```python
from build123d import *

# Parameters (mm, degrees)
SZKIC1_R                        = 5
DODANIE_WYCI_GNI_CIE1_DEPTH     = 18
WYTNIJ_WYCI_GNI_CIE1_DEPTH      = 5
WYTNIJ_WYCI_GNI_CIE1_DEPTH_BACK = 5
WYTNIJ_WYCI_GNI_CIE2_DEPTH      = 5
WYTNIJ_WYCI_GNI_CIE2_DEPTH_BACK = 3
SZKIC3_W                        = 2.5
SZKIC3_H                        = 5.64
WYTNIJ_WYCI_GNI_CIE3_REACH      = 21.339
SZKIC4_R                        = 1.6
WYTNIJ_WYCI_GNI_CIE4_DEPTH      = 2.5


with BuildPart() as part:
    # Szkic1 → Dodanie-wyciągnięcie1 (new body)
    with BuildSketch(Plane.XY):
        Circle(SZKIC1_R)
    extrude(amount=DODANIE_WYCI_GNI_CIE1_DEPTH)

    # Szkic2 → Wytnij-wyciągnięcie1 (cut, two sides: drawn at the far end of the back side and taken through both)
    with BuildSketch(Plane(origin=(0, 0, 0), x_dir=(1, 0, 0), z_dir=(0, 1, 0)).offset(-WYTNIJ_WYCI_GNI_CIE1_DEPTH_BACK)):
        Polygon((-5, -18), (5, -18), (-5, -8), align=None)
    extrude(amount=WYTNIJ_WYCI_GNI_CIE1_DEPTH + WYTNIJ_WYCI_GNI_CIE1_DEPTH_BACK, mode=Mode.SUBTRACT)

    # Szkic3 → Wytnij-wyciągnięcie2 (cut, two sides: drawn at the far end of the back side and taken through both)
    with BuildSketch(Plane(origin=(0, 0, 0), x_dir=(0, 0, -1), z_dir=(1, 0, 0)).offset(-WYTNIJ_WYCI_GNI_CIE2_DEPTH_BACK)):
        with Locations((-3.25, 0)):
            Rectangle(SZKIC3_W, SZKIC3_H)
    extrude(amount=WYTNIJ_WYCI_GNI_CIE2_DEPTH + WYTNIJ_WYCI_GNI_CIE2_DEPTH_BACK, mode=Mode.SUBTRACT)

    # Szkic4 → Wytnij-wyciągnięcie3 (cut, up to next)
    with BuildSketch(Plane(origin=(0, 0, 0), x_dir=(-1, 0, 0), z_dir=(0, 0, -1)), mode=Mode.PRIVATE) as wytnij_wyci_gni_cie3_sk1:
        Circle(SZKIC4_R)
    wytnij_wyci_gni_cie3_tool1 = extrude(wytnij_wyci_gni_cie3_sk1.sketch, amount=-WYTNIJ_WYCI_GNI_CIE3_REACH, mode=Mode.PRIVATE) & part.part
    add(wytnij_wyci_gni_cie3_tool1.solids().sort_by_distance((0, 0, 0))[0], mode=Mode.SUBTRACT)

    # Szkic5 → Wytnij-wyciągnięcie4 (cut)
    with BuildSketch(Plane.XY.offset(2)):
        Polygon((-3, -2.82), (-3, 2.82), (-4.333128401, 0), align=None)
    extrude(amount=WYTNIJ_WYCI_GNI_CIE4_DEPTH, mode=Mode.SUBTRACT)


solid = part.part
```
Design review of the part built by this model. Coordinates are the model's own, in mm. A direction names the side the tool comes from. Give positions to 0.01 mm unless a question says otherwise; leave off trailing zeros. Order: outer loops, then holes, each group sorted by start corner. A loop starts at its lowest first (then second) coordinate and runs counter-clockwise, first axis right, second up. Notation, with made-up numbers: (86.25, -11.75) -> (137.25, -11.75) arc R23 cw to (137.25, 20.25) -> close; hole circle Ø4 at (12, -2). An arc over 180 degrees is marked (long way). Write item = value, one per line. Start each with the question number.
(1) For pin 1 (4 mm diameter, centred on x = -2.5, z = 10, fed in from +Y); pin 2 (3 mm diameter, centred on x = 2, y = 0, fed in from +Z); pin 3 (3.5 mm diameter, centred on x = 0, y = 0, fed in from +Z), all flat-tipped, find the tip position at first contact; note any pin that passes through.
(2) We need section C-C on x = 0. Write out the cut boundary in (y, z).
(3) We need section D-D on z = 4. Write out the cut boundary in (x, y).
(4) For faces 1 (the face through (1, 2.82, 3)), 2 (the face through (1.27, -0.97, 0.99)), 3 (the face through (4.77, 1.5, 6.87)), list the 3-axis set-ups (+Z, -Z, +X, -X, +Y, -Y) from which the entire face can be reached by the end or side of a thin tool; tool diameter is ignored.
(5) We need section A-A on x = 3. Write out the cut boundary in (y, z).
(6) We need section B-B on y = 1. Write out the cut boundary in (x, z).
(7) Mouldability with a two-part tool opening along Z and no side actions: class faces 4 (the face through (2, 0, 0)), 5 (the face through (1, -2.82, 3)), 6 (the face through (0, 0, 4.5)), 7 (the face through (0, 0, 13)) as +Z half, -Z half, draft (parallel to the pull), parting line (faces both ways), or undercut.
(8) To check wall thickness, follow line 1 along Y through (x, z) = (0, 0.95); line 2 along Y through (x, z) = (-2, 3); line 3 along Z through (x, y) = (2, -2.75). State the ranges of each line that lie inside material, in increasing order.
Numbers:
q1.pin_1 = 4.97
q1.pin_2 = 16.5
q1.pin_3 = 14.75
q2.outline = (-5, 0) -> (-1.6, 0) -> (-1.6, 2) -> (-2.82, 2) -> (-2.82, 4.5) -> (2.82, 4.5) -> (2.82, 2) -> (1.6, 2) -> (1.6, 0) -> (5, 0) -> (5, 13) -> (-5, 13) -> close
q3.outline = (-4.33, 0) -> (-3, 2.82) -> (4.13, 2.82) arc R5 ccw (long way) to (4.13, -2.82) -> (-3, -2.82) -> close
q4.face_1 = +X
q4.face_2 = -Z
q4.face_3 = +Z, -Z
q5.outline = (-4, 0) -> (4, 0) -> (4, 16) -> (-4, 16) -> close; hole (-2.82, 2) -> (2.82, 2) -> (2.82, 4.5) -> (-2.82, 4.5) -> close
q6.outline = (-4.9, 0) -> (-1.25, 0) -> (-1.25, 2) -> (-3.86, 2) -> (-3.86, 4.5) -> (4.9, 4.5) -> (4.9, 17.9) -> (-4.9, 8.1) -> close; (1.25, 0) -> (4.9, 0) -> (4.9, 2) -> (1.25, 2) -> close
q7.face_4 = -Z half
q7.face_5 = undercut
q7.face_6 = undercut
q7.face_7 = +Z half
q8.line_1 = -5 to -1.6, 1.6 to 5
q8.line_2 = -4.58 to -2.82, 2.82 to 4.58
q8.line_3 = 0 to 2, 4.5 to 15
